The listing builds one solid part. Answer for the finished solid, in the listing's coordinates (mm). Coordinates: 2 decimals unless noted, no trailing zeros. One line per item, written item: value. Start each with the question number.
Q1. The part is cut by section A-A on y = 1.3. Give the number of separate pieces and of enclosed holes in the cut face, then the cut area to 3 significant figures.
Q2. Straight lines are drawn through the part: line 1 along X through (y, z) = (1.55, 32); line 2 along Z through (x, y) = (-27, 1.15); line 3 along Z through (x, y) = (38.1, 1.6). For each, find the intervals that lie inside material, in ascending order. Write a range as [from, to].
Q3. Each of these flat-tipped pins is pushed along its axis until it touches: pin 1 Ø2 at (x, z) = (72.5, -33) entering from -Y; pin 2 Ø1.6 at (y, z) = (1, 25.5) entering from -X; pin 3 Ø1 at (y, z) = (1, 27.5) entering from +X; pin 4 Ø1 at (y, z) = (2, 28.5) entering from -X. Where does it stop, or does it pass through?
Autodesk Inventor part; units mm, degrees
ref_plane "YZ Plane" through (0, 0, 0) normal (1, 0, 0) x (0, 1, 0)
ref_plane "XZ Plane" through (0, 0, 0) normal (0, 1, 0) x (-1, 0, 0)
ref_plane "XY Plane" through (0, 0, 0) normal (0, 0, 1) x (1, 0, 0)
sketch "Sketch1" plane through (0, 0, 0) normal (0, 1, 0) x (-1, 0, 0)
  line L0 (101.6, 38.1) -> (-101.6, 38.1) construction
  line L1 (-101.6, 38.1) -> (-101.6, -38.1) construction
  line L2 (-101.6, -38.1) -> (101.6, -38.1) construction
  line L3 (101.6, -38.1) -> (101.6, 38.1) construction
  line L4 (101.6, 38.1) -> (-101.6, -38.1) construction
  line L5 (-101.6, 38.1) -> (101.6, -38.1) construction
  line L6 (-28.575, 66.675) -> (28.575, 66.675) construction
  line L7 (28.575, 66.675) -> (28.575, 9.525)
  line L8 (28.575, 9.525) -> (-28.575, 9.525)
  line L9 (-28.575, 9.525) -> (-28.575, 66.675)
  line L10 (-28.575, 66.675) -> (28.575, 9.525) construction
  line L11 (28.575, 66.675) -> (-28.575, 9.525) construction
  circle A0 centre (-38.1, 50.8) radius 3.175
  line L12 (0, 38.1) -> (0, -38.1) construction
  circle A1 centre (-38.1, 50.8) radius 9.525
  line L13 (-38.1, 60.325) -> (-28.575, 60.325)
  circle A2 centre (38.1, 50.8) radius 3.175
  circle A3 centre (38.1, 50.8) radius 9.525
  line L14 (38.1, 60.325) -> (28.575, 60.325)
  circle A4 centre (-76.2, -38.1) radius 1.7526
  circle A5 centre (-95.25, 3.175) radius 1.7526
  circle A6 centre (76.2, -38.1) radius 1.7526
  circle A7 centre (95.25, 3.175) radius 1.7526
  line L15 (-101.6, -38.1) -> (-101.6, 6.35)
  line L16 (-101.6, 6.35) -> (-44.4797, 57.8728)
  line L17 (101.6, -38.1) -> (101.6, 6.35)
  line L18 (101.6, 6.35) -> (44.4797, 57.8728)
  line L19 (-42.6417, 42.4275) -> (-87.975, 1.5367)
  line L20 (-87.975, 1.5367) -> (-87.975, -38.1)
  line L21 (87.975, -38.1) -> (87.975, 1.5367)
  line L22 (87.975, 1.5367) -> (42.6417, 42.4275)
  line L23 (0, -38.1) -> (-95.25, -38.1) construction
  line L24 (0, -38.1) -> (95.25, -38.1) construction
  circle A8 centre (-60.325, 35.0287) radius 1.7526
  circle A9 centre (-33.3375, 31.75) radius 1.7526
  line L25 (-38.1, 0) -> (-38.1, 41.275)
  line L26 (-38.1, 0) -> (0, 0) construction
  circle A10 centre (60.325, 35.0287) radius 1.7526
  circle A11 centre (33.3375, 31.75) radius 1.7526
  line L27 (38.1, 0) -> (38.1, 41.275)
  line L28 (38.1, 0) -> (0, 0) construction
  line L29 (-87.975, 0) -> (-65.115, 0)
  line L30 (-65.115, 0) -> (-65.115, -31.75)
  line L31 (-65.115, -31.75) -> (-87.975, -31.75)
  line L32 (-101.6, -38.1) -> (101.6, -38.1) construction
  line L33 (101.6, -38.1) -> (101.6, 19.05)
  line L34 (101.6, 19.05) -> (-101.6, 19.05) construction
  line L35 (-101.6, 19.05) -> (-101.6, -38.1)
  line L36 (-101.6, 19.05) -> (-87.5203, 19.05) construction
  line L37 (87.5203, 19.05) -> (101.6, 19.05) construction
  circle A12 centre (-38.1, 0) radius 3.175 construction
  circle A13 centre (-38.1, 0) radius 6.35 construction
  circle A14 centre (38.1, 0) radius 3.175 construction
  circle A15 centre (38.1, 0) radius 6.35 construction
  circle A16 centre (28.575, 9.525) radius 1.7526
  circle A17 centre (28.575, 9.525) radius 4.7625
  arc A18 (17.0773, 9.525) -> (28.575, 21.0227) centre (17.0773, 21.0227) ccw
  circle A19 centre (-28.575, 9.525) radius 1.7526
  circle A20 centre (-28.575, 9.525) radius 4.7625
  arc A21 (-28.575, 21.0227) -> (-17.0773, 9.525) centre (-17.0773, 21.0227) ccw
  arc A22 (31.4325, 5.715) -> (38.1, 19.05) centre (21.4312, 19.05) ccw
  arc A23 (-38.1, 19.05) -> (-31.4325, 5.715) centre (-21.4312, 19.05) ccw
  line L38 (-61.94, -38.1) -> (-61.94, 25.0204)
  line L39 (87.975, 0) -> (65.115, 0)
  line L40 (65.115, 0) -> (65.115, -31.75)
  line L41 (65.115, -31.75) -> (87.975, -31.75)
  line L42 (61.94, -38.1) -> (61.94, 25.0204)
  line L43 (-28.575, 4.7625) -> (28.575, 4.7625)
  line L44 (101.6, -31.75) -> (-101.6, -31.75)
  line L45 (-101.6, -31.75) -> (-101.6, -44.45) construction
  line L46 (-101.6, -44.45) -> (101.6, -44.45)
  line L47 (101.6, -44.45) -> (101.6, -31.75) construction
  circle A24 centre (0, -38.1) radius 1.7526
  circle A25 centre (38.1, -38.1) radius 1.7526
  circle A26 centre (-38.1, -38.1) radius 1.7526
  line L48 (101.6, -38.1) -> (76.2, -44.45)
  line L49 (-101.6, -38.1) -> (-76.2, -44.45)
  line L50 (76.2, -38.1) -> (76.2, -44.45) construction
  line L51 (-76.2, -38.1) -> (-76.2, -44.45) construction
  line L52 (59.1924, 41.2769) -> (32.488, 36.4361)
  circle A27 centre (60.325, 35.0287) radius 6.35
  circle A28 centre (33.3375, 31.75) radius 4.7625
  line L53 (-59.1924, 41.2769) -> (-32.488, 36.4361)
  circle A29 centre (-60.325, 35.0287) radius 6.35
  circle A30 centre (-33.3375, 31.75) radius 4.7625
  line L54 (-87.975, 0) -> (-65.115, 0)
  line L55 (-65.115, 0) -> (-65.115, -3.175)
  line L56 (-65.115, -3.175) -> (-87.975, -3.175)
  line L57 (-87.975, -3.175) -> (-87.975, 0)
  line L58 (-65.115, -15.875) -> (-87.975, -15.875) construction
  line L59 (-65.115, -28.575) -> (-87.975, -28.575)
  line L60 (-84.8, -38.1) -> (-84.8, 0.1248)
  line L61 (65.115, -3.175) -> (87.975, -3.175)
  line L62 (65.115, -15.875) -> (87.975, -15.875) construction
  line L63 (65.115, -28.575) -> (87.975, -28.575)
  line L64 (84.8, -38.1) -> (84.8, 0.1248)
  point P0 (28.575, 38.1)
  point P1 (-28.575, 38.1)
  point P2 (28.575, 60.325)
  point P3 (44.4797, 57.8728)
  point P4 (101.6, -15.875)
  point P5 (38.1, 41.275)
  point P6 (-87.975, -31.75)
  point P7 (-101.6, 6.35)
  point P8 (101.6, 6.35)
  point P9 (31.75, 0)
  point P10 (38.1, 6.35)
  point P11 (-38.1, 6.35)
  point P12 (-31.75, 0)
  point P13 (87.975, 0)
  point P14 (61.94, 25.0204)
  point P15 (-17.0773, 9.525)
  point P16 (-28.575, 21.0227)
  point P17 (-38.1, 19.05)
  point P18 (-31.4325, 5.715)
  point P19 (-21.8502, 0)
  point P20 (21.8502, 0)
  point P21 (-25.2074, 12.8926)
  point P22 (-28.575, 14.2875)
  point P23 (-23.8125, 9.525)
  point P24 (-28.575, 50.8)
  point P25 (25.2074, 12.8926)
  point P26 (28.575, 14.2875)
  point P27 (23.8125, 9.525)
  point P28 (28.575, 50.8)
  point P29 (26.8224, 9.525)
  point P30 (28.575, 11.2776)
  point P31 (61.94, -31.75)
  point P32 (-61.94, -31.75)
  point P33 (-28.575, 31.75)
  point P34 (-64.5781, 39.7439)
  point P35 (64.5781, 39.7439)
  point P36 (28.575, 31.75)
  point P37 (-84.8, -3.175)
  point P38 (-84.8, -28.575)
  point P39 (84.8, -3.175)
  point P40 (84.8, -28.575)
  point P41 (-101.6, -31.75)
  point P42 (-56.0719, 30.3135)
  point P43 (56.0719, 30.3135)
  point P44 (46.4735, 38.9713)
  point P45 (-46.4735, 38.9713)
  point P46 (-28.575, 11.2776)
  point P47 (-26.8224, 9.525)
  dimension "d0" = 203.2
  dimension "d1" = 76.2
  dimension "d4" = 57.15
  dimension "d6" = 6.35
  dimension "d7" = 38.1
  dimension "d8" = 19.05
  dimension "d10" = 3.5052
  dimension "d11" = 3.5052
  dimension "d12" = 0
  dimension "d14" = 25.4
  dimension "d15" = 6.35
  dimension "d20" = 50.8
  dimension "d21" = 41.275
  dimension "d22" = 44.45
  dimension "d24" = 12.7
  dimension "d25" = 13.625
  dimension "d26" = 12.7
  dimension "d27" = 13.625
  dimension "d31" = 3.5052
  dimension "d32" = 3.5052
  dimension "d33" = 6.35
  dimension "d34" = 31.75
  dimension "d35" = 4.7625
  dimension "d36" = 22.225
  dimension "d37" = 9.525
  dimension "d39" = 31.75
  dimension "d40" = 6.35
  dimension "d42" = 57.15
  dimension "d43" = 6.35
  dimension "d44" = 9.525
  dimension "d45" = 9.525
  dimension "d46" = 12.7
  dimension "d104" = 3.5052
  dimension "d105" = 9.525
  dimension "d106" = 3.175
  dimension "d107" = 22.86
  dimension "d123" = 88.9
  dimension "d124" = 12.7
  dimension "d125" = 3.5052
  dimension "d126" = 3.5052
  dimension "d127" = 38.1
  dimension "d128" = 28.575
  dimension "d129" = 3.175
  dimension "d130" = 3.175
extrude "Extrusion1" add sketch "Sketch1" along normal blind 3.175 contours A28 L27 A22 A17 L7 | A28 | L7 A17 A18 | L52 L27 A28 | L27 L52 L22 L42 L44 L38 L19 L53 L25 A23 A20 L43 A17 A22 | L18 L17 L44 L21 L22 A27 | A27 | A17 L8 A16 L7 | L7 A16 L8 A17 | A17 L8 A18 | L52 A27 L22 | A17 L43 A20 L8 | L17 L48 L46 L49 L15 L44 L31 L41 | L8 A20 A21 | L22 L21 L39 L40 L44 L42 | L41 L64 L63 L21 | A20 L9 A19 L8 | L8 A19 L9 A20 | A20 L9 A21 | L63 L64 L61 L21 | L41 L40 L63 L64 | A23 L25 A30 L9 A20 | L21 L61 L64 L39 | L44 L30 L29 L20 L19 L38 | L63 L40 L61 L64 | A30 | L64 L61 L40 L39 | L19 L20 L44 L15 L16 A29 | L31 L60 L59 L30 | L25 L53 A30 | A29 L53 L19 | A29 | L59 L60 L56 L30 | L31 L20 L59 L60 | L29 L60 L56 L20 | L56 L60 L29 L30 | L59 L20 L56 L60
fillet "Fillet1" radius 6.35 6 edges at (101.6, 1.5875, -38.1) (101.6, 1.5875, 6.35) (-101.6, 1.5875, 6.35) (76.2, 1.5875, -44.45) (-76.2, 1.5875, -44.45) (-101.6, 1.5875, -38.1)
equation "\"d35\" = 0.5 * d37"
properties part number "Chassis" material "UHMW, White"
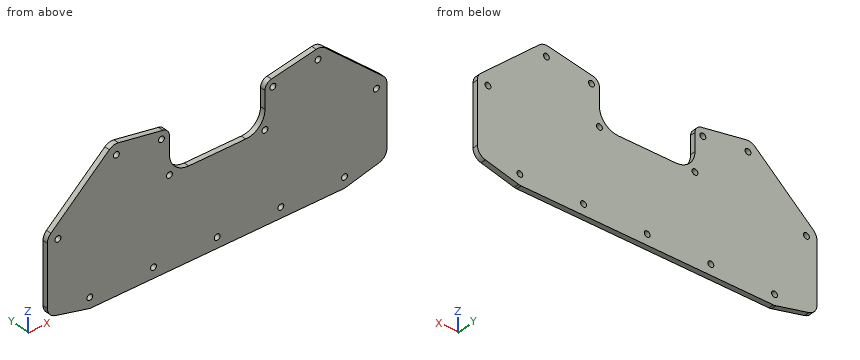
Output:
1. separate pieces: 1
1. enclosed holes: 13
1. area: 13,800 mm^2
2. line 1: x = [-73.16, -35.07], [-31.6, -28.58], [28.58, 31.6], [35.07, 73.16]
2. line 2: z = [-44.45, 8.76], [10.29, 15.21]
2. line 3: z = [-44.45, -39.85], [-36.35, 37.45]
3. pin 1: stops at y = 0
3. pin 2: stops at x = -81.26
3. pin 3: stops at x = 78.71
3. pin 4: stops at x = -77.6
